Study the drawing (mm; zero at the part's minimum x, y, z) and answer. A direction names the side the tool comes from. Round coordinates to 2 decimals unless told otherwise and drop trailing zeros. Write each loop counter-clockwise with the first axis right and the second up, starting at its lowest first coordinate (ties: lowest second). Pieces come first, ordered by that corner, then holes.
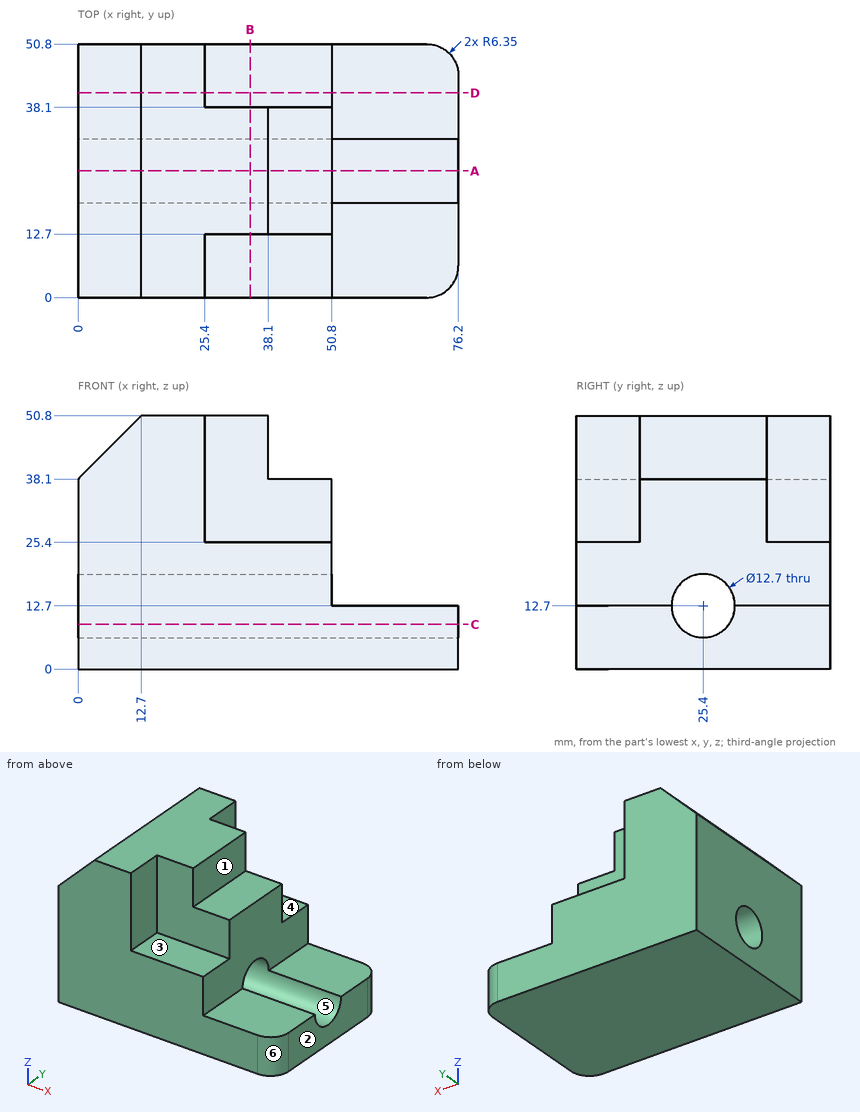
Q1. Find section B-B (x = 34.5). Determine the outline of the cut face in (y, z), plus the area to 3 significant figures.
Q2. Find the intervals of material crossed by L1, parallel to Z at x = 21.5, y = 25.4; L2, parallel to Z at x = 39.5, y = 25.4; L3, parallel to Z at x = 68, y = 5, in increasing order.
Q3. A tool of negligible diameter and unlimited length cuts with its end or side. For the marked faces 1, 2 and 3, from which of +Z, -Z, +X, -X, +Y, -Y can it reach the whole face along a straight path? Write none if from no direction.
Q4. Find section A-A (y = 25.4). Determine the outline of the cut face in (x, z), plus the area to 3 significant figures.
Q5. Given pin 1 (4 mm diameter, centred on y = 6.5, z = 44, fed in from +X); pin 2 (5.5 mm diameter, centred on x = 60, y = 9.5, fed in from +Z); pin 3 (10 mm diameter, centred on x = 40, y = 6, fed in from +Z), each flat-ended and moving along its own axis, determine where each tip first touches the part or whether it passes through.
Q6. Find section C-C (z = 9). Determine the outline of the cut face in (x, y), plus the area to 3 significant figures.
Q7. Find section D-D (y = 41). Determine the outline of the cut face in (x, z).
Q8. The mould has two halves that part along Z. Classify the marked faces 4, 5 and 6: +Z half, -Z half, draft (parallel to the pull), parting line (faces both ways), or undercut.
Report:
1. outline: (0, 0) - (50.8, 0) - (50.8, 25.4) - (38.1, 25.4) - (38.1, 50.8) - (12.7, 50.8) - (12.7, 25.4) - (0, 25.4) - close; hole circle Ø12.7 at (25.4, 12.7)
1. area: 1,810 mm2
2. L1: z = 0 to 6.35, 19.05 to 50.8
2. L2: z = 0 to 6.35, 19.05 to 38.1
2. L3: z = 0 to 12.7
3. face 1: +Z, +X, +Y, -Y
3. face 2: +Z, -Z, +X, +Y, -Y
3. face 3: +Z, +X, -Y
4. outline: (0, 0) - (76.2, 0) - (76.2, 6.35) - (0, 6.35) - close; (0, 19.05) - (50.8, 19.05) - (50.8, 38.1) - (38.1, 38.1) - (38.1, 50.8) - (12.7, 50.8) - (0, 38.1) - close
4. area: 1,850 mm2
5. pin 1: stops at x = 25.4
5. pin 2: stops at z = 12.7
5. pin 3: stops at z = 25.4
6. outline: (0, 0) - (69.85, 0) arc R6.35 ccw to (76.2, 6.35) - (76.2, 20.24) - (0, 20.24) - close; (0, 30.56) - (76.2, 30.56) - (76.2, 44.45) arc R6.35 ccw to (69.85, 50.8) - (0, 50.8) - close
6. area: 3,070 mm2
7. outline: (0, 0) - (76.2, 0) - (76.2, 12.7) - (50.8, 12.7) - (50.8, 25.4) - (25.4, 25.4) - (25.4, 50.8) - (12.7, 50.8) - (0, 38.1) - close
8. face 4: +Z half
8. face 5: undercut
8. face 6: draft
